Design review of the part built by this model. Coordinates are the model's own, in mm. A direction names the side the tool comes from. Round coordinates to 2 decimals unless told otherwise and drop trailing zeros. Write each loop counter-clockwise with the first axis right and the second up, starting at its lowest first coordinate (ties: lowest second). Pieces come first, ordered by that corner, then holes. Notation, with made-up numbers: (-1, 42) - (56, 42) arc R19 ccw to (56, 69) - close; hole circle Ø1 at (41.25, 82.25). An arc over 180 degrees is marked (long way). Use one line per item in the form item = value.
```python
from build123d import *

# Parameters (mm, degrees)
BOSS_EXTRUDE1_DEPTH      = 35
DRAFT3_START             = 66.714465374
DRAFT3_OUTLINE_W         = 72
DRAFT3_OUTLINE_H         = 84
DRAFT3_DEPTH             = 6.038326985
BOSS_EXTRUDE3_DEPTH      = 10
BOSS_EXTRUDE3_DEPTH_BACK = 10
SKETCH8_R                = 25


# Read off the part's stored shape, not the designer's step: Draft3
with BuildPart() as part:
    # Sketch3 for Loft2 → Loft2 section 0
    with BuildSketch(Plane(origin=(0, 0, 0), x_dir=(1, 0, 0), z_dir=(0, 1, 0))):
        with BuildLine():
            # circular arc as an exact rational Bezier (weights 1, cos(half-angle), 1)
            Bezier((-34.641016151, 20), (-23.094010767, 39.999999999), (0, 40), weights=[1, 0.866025404, 1])
            Bezier((0, 40), (23.094010767, 39.999999999), (34.641016151, 20), weights=[1, 0.866025404, 1])
            Bezier((34.641016151, 20), (46.188021536, 0), (34.641016151, -20), weights=[1, 0.866025404, 1])
            Bezier((34.641016151, -20), (23.094010767, -39.999999999), (0, -40), weights=[1, 0.866025404, 1])
            Bezier((0, -40), (-23.094010767, -39.999999999), (-34.641016151, -20), weights=[1, 0.866025404, 1])
            Bezier((-34.641016151, -20), (-46.188021536, 0), (-34.641016151, 20), weights=[1, 0.866025404, 1])
        make_face()
    # Sketch4 → Loft2 section 1
    with BuildSketch(Plane(origin=(0, 35, 0), x_dir=(-1, 0, 0), z_dir=(0, -1, 0))):
        with BuildLine():
            Line((34.641016151, 20), (0, 40))
            Line((0, 40), (-34.641016151, 20))
            Line((-34.641016151, 20), (-34.641016151, -20))
            Line((-34.641016151, -20), (0, -40))
            Line((0, -40), (34.641016151, -20))
            Line((34.641016151, -20), (34.641016151, 20))
        make_face()
    loft()

    # Sketch7 → Boss-Extrude1 (add)
    with BuildSketch(Plane(origin=(0, 35, 0), x_dir=(1, 0, 0), z_dir=(0, 1, 0))):
        Polygon((-34.641016151, 20), (-34.641016151, -20), (0, -40), (34.641016151, -20), (34.641016151, 20), (0, 40), align=None)
    extrude(amount=BOSS_EXTRUDE1_DEPTH)

    # Draft3 outline → Draft3 (cut)
    with BuildSketch(Plane(origin=(0, 0, 0), x_dir=(0.9961946980917452, -0.08715574274766182, 0), z_dir=(0.08715574274766182, 0.9961946980917452, 0)).offset(DRAFT3_START)):
        with Locations((-6, 0)):
            Rectangle(DRAFT3_OUTLINE_W, DRAFT3_OUTLINE_H)
    extrude(amount=DRAFT3_DEPTH, mode=Mode.SUBTRACT)

    # Sketch8 → Boss-Extrude3 (add, two sides: drawn at the far end of the back side and taken through both)
    with BuildSketch(Plane(origin=(0, 70, 0), x_dir=(1, 0, 0), z_dir=(0, 1, 0)).offset(-BOSS_EXTRUDE3_DEPTH_BACK)):
        with Locations(Location((0, 0, 0), (0, 0, 180))):
            Circle(SKETCH8_R)
    extrude(amount=BOSS_EXTRUDE3_DEPTH + BOSS_EXTRUDE3_DEPTH_BACK)


solid = part.part
```
Q1. To check wall thickness, follow line 1 along X through (y, z) = (45.5, 14); line 2 along X through (y, z) = (16.5, 25); line 3 along Z through (x, y) = (-1, 11). State the ranges of each line that lie inside material, in increasing order. Write a range as from..to.
Calculated:
line_1 = -34.64..34.64
line_2 = -29.3..29.3
line_3 = -39.83..39.83
Q2. Machinability: for faces 1 (the flat face through (34.641, 49, 0)), 2 (the flat face through (17.56, 50.76, -29.86)), 3 (the flat face through (-34.641, 52, 0)), 4 (the flat face through (-17.56, 52.26, 29.86)), which of the approach directions +Z, -Z, +X, -X, +Y, -Y give a long, thin tool a straight path to every point of the face, cutting with its end or side? Answer none if there is none.
Calculated:
face_1 = +Z, -Z, +X, +Y
face_2 = -Z, +X, +Y
face_3 = +Z, -Z, -X, +Y
face_4 = +Z, -X, +Y
Q3. We need section A-A on y = 53. Write out the cut boundary in (x, z).
Calculated:
outline = (-34.64, -20) - (0, -40) - (34.64, -20) - (34.64, 20) - (0, 40) - (-34.64, 20) - close
Q4. For P1, Ø4, axis at y = 31, z = -16, coming from the +X side; P2, Ø3, axis at x = 17.5, z = 27.5, coming from the +Y side; P3, Ø8, axis at y = 55, z = 12.5, coming from the +X side, all flat-tipped, find the tip position at first contact; note any pin that passes through.
Calculated:
P1 = 35.02
P2 = 65.57
P3 = 34.64
